```python
from build123d import *

# Parameters (mm, degrees)
SKETCH_1_R          = 16
EXTRUDE_1_DEPTH     = 8
SKETCH_2_R          = 2
CUT_EXTRUDE_1_DEPTH = 6
CUT_EXTRUDE_START   = -6
SKETCH_3_R          = 2
CUT_EXTRUDE_2_DEPTH = 6
FILLET_1_R          = 2
FILLET_2_R          = 2
SKETCH_4_R          = 16
SKETCH_4_R_2        = 12.5
EXTRUDE_2_DEPTH     = 3


with BuildPart() as part:
    # 草图1 → 凸台-拉伸1 (new body)
    with BuildSketch(Plane.XY):
        with BuildLine():
            Line((-26, 23.2), (26, 23.2))
            Line((26, 23.2), (26, 17.2))
            Line((26, 17.2), (10.205880658, 17.2))
            ThreePointArc((10.205880658, 17.2), (20, 0), (10.205880658, -17.2))
            Line((10.205880658, -17.2), (26, -17.2))
            Line((26, -17.2), (26, -23.2))
            Line((26, -23.2), (-26, -23.2))
            Line((-26, -23.2), (-26, -17.2))
            Line((-26, -17.2), (-10.205880658, -17.2))
            ThreePointArc((-10.205880658, -17.2), (-20, 0), (-10.205880658, 17.2))
            Line((-10.205880658, 17.2), (-26, 17.2))
            Line((-26, 17.2), (-26, 23.2))
        make_face()
        Circle(SKETCH_1_R, mode=Mode.SUBTRACT)
    extrude(amount=EXTRUDE_1_DEPTH)

    # 草图2 → 切除-拉伸1 (cut)
    with BuildSketch(Plane(origin=(0, 23.2, 0), x_dir=(1, 0, 0), z_dir=(0, 1, 0))):
        with Locations(Location((-20, -4, 0), (0, 0, 270))):
            Circle(SKETCH_2_R)
        with Locations(Location((20, -4, 0), (0, 0, 90))):
            Circle(SKETCH_2_R)
    extrude(amount=-CUT_EXTRUDE_1_DEPTH, mode=Mode.SUBTRACT)

    # 草图3 → 切除-拉伸2 (cut)
    with BuildSketch(Plane.XZ.offset(23.2).offset(CUT_EXTRUDE_START)):
        with Locations(Location((20, 4, 0), (0, 0, 270))):
            Circle(SKETCH_3_R)
        with Locations(Location((-20, 4, 0), (0, 0, 90))):
            Circle(SKETCH_3_R)
    extrude(amount=CUT_EXTRUDE_2_DEPTH, mode=Mode.SUBTRACT)

    # 圆角1
    fillet_1_edges = [part.edges().sort_by_distance(p)[0] for p in [
        (-10.205880658, -17.2, 4),
        (-10.205880658, 17.2, 4),
        (10.205880658, 17.2, 4),
        (10.205880658, -17.2, 4),
    ]]
    fillet(fillet_1_edges, radius=FILLET_1_R)

    # 圆角2
    fillet_2_edges = [part.edges().sort_by_distance(p)[0] for p in [
        (-26, -17.2, 4),
        (-26, 17.2, 4),
        (26, 17.2, 4),
        (26, -17.2, 4),
    ]]
    fillet(fillet_2_edges, radius=FILLET_2_R)

    # 草图4 → 凸台-拉伸2 (add)
    with BuildSketch(Plane(origin=(0, 0, 0), x_dir=(-1, 0, 0), z_dir=(0, 0, -1))):
        Circle(SKETCH_4_R)
        Circle(SKETCH_4_R_2, mode=Mode.SUBTRACT)
    extrude(amount=-EXTRUDE_2_DEPTH)


solid = part.part
```
Can you work these out from the model? Positions are in its coordinate system, mm. A direction names the side the tool comes from. Round coordinates to 2 decimals unless told otherwise and drop trailing zeros. Order: outer loops, then holes, each group sorted by start corner. A loop starts at its lowest first (then second) coordinate and runs counter-clockwise, first axis right, second up. Notation, with made-up numbers: (-29.5, 68) -> (18.5, 68) arc R25 cw to (18.5, 101) -> close; hole circle Ø7 at (63.5, -38). An arc over 180 degrees is marked (long way). Return JSON: item names as keys, results as strings. Group by question number.
1. If we section it at B-B, the plane y = 0: Write out the boundary of the cut face in (x, z).
2. If we section it at A-A, the plane x = 0: Write out the boundary of the cut face in (y, z), then the cut area to 3 significant figures.
3. If we section it at C-C, the plane z = 7: Write out the boundary of the cut face in (x, y), then the cut area to 3 significant figures.
4. We'd pull the mould along Y, two halves only. Please class faces 1 (the face through (-18, 20, 4)), 2 (the face through (0, 23.2, 4)), 3 (the face through (20, 0, 4)): released by +Y, released by -Y, zero draft, split by the parting line, or undercut.
5. If we section it at D-D, the plane y = -20: Write out the boundary of the cut face in (x, z), then the cut area to 3 significant figures.
6. I need wall thicknesses on line 1 (X direction, y = 20.9, z = 4); line 2 (Y direction, x = 0.5, z = 1.25); line 3 (Y direction, x = 18, z = 5.25). Which ranges of each line are inside material? Lowest first, please. Write a range as [from, to].
7. Which directions (+Z, -Z, +X, -X, +Y, -Y) give clear straight access to the entire face, cutting with the end or side of a thin tool? Please do faces 4 (the face through (25.43, -17.8, 4.06)), 5 (the face through (10, -8, 3)), 6 (the face through (-25.4, 17.77, 4.06)).
8. Will these pins go through, and if not, where does the flat tip stop? pin 1 (3.5 mm diameter, centred on x = 20, z = 4, fed in from -Y); pin 2 (9.5 mm diameter, centred on x = 3.5, y = 5, fed in from +Z).
Output values:
{
 "1": {"outline": "(-20, 0) -> (-12.5, 0) -> (-12.5, 3) -> (-16, 3) -> (-16, 8) -> (-20, 8) -> close; (12.5, 0) -> (20, 0) -> (20, 8) -> (16, 8) -> (16, 3) -> (12.5, 3) -> close"},
 "2": {"outline": "(-23.2, 0) -> (-12.5, 0) -> (-12.5, 3) -> (-16, 3) -> (-16, 8) -> (-23.2, 8) -> close; (12.5, 0) -> (23.2, 0) -> (23.2, 8) -> (16, 8) -> (16, 3) -> (12.5, 3) -> close", "area": "136 mm²"},
 "3": {"outline": "(-26, -23.2) -> (26, -23.2) -> (26, -19.2) arc R2 ccw to (24, -17.2) -> (15.9, -17.2) arc R2 cw to (14.46, -13.82) arc R20 ccw to (14.46, 13.82) arc R2 cw to (15.9, 17.2) -> (24, 17.2) arc R2 ccw to (26, 19.2) -> (26, 23.2) -> (-26, 23.2) -> (-26, 19.2) arc R2 ccw to (-24, 17.2) -> (-15.9, 17.2) arc R2 cw to (-14.46, 13.82) arc R20 ccw to (-14.46, -13.82) arc R2 cw to (-15.9, -17.2) -> (-24, -17.2) arc R2 ccw to (-26, -19.2) -> close; hole circle Ø32 at (0, 0)", "area": "1,020 mm²"},
 "4": {"face 1": "zero draft", "face 2": "released by +Y", "face 3": "undercut"},
 "5": {"outline": "(-26, 0) -> (26, 0) -> (26, 8) -> (-26, 8) -> close; hole circle Ø4 at (-20, 4); hole circle Ø4 at (20, 4)", "area": "391 mm²"},
 "6": {"line 1": "[-26, -22], [-18, 18], [22, 26]", "line 2": "[-23.2, -12.49], [12.49, 23.2]", "line 3": "[-23.2, -17.2], [-8.72, 8.72], [17.2, 23.2]"},
 "7": {"face 4": "+Z, -Z, +X", "face 5": "+Z", "face 6": "+Z, -Z, -X"},
 "8": {"pin 1": "y = -8.18", "pin 2": "through"}
}
